from build123d import *

# Parameters (mm, degrees)
SKETCH2_R           = 4
SKETCH2_R_2         = 1.5
BOSS_EXTRUDE1_DEPTH = 5


with BuildPart() as part:
    # Sketch2 → Boss-Extrude1 (new body)
    with BuildSketch(Plane(origin=(0, 0, 0), x_dir=(1, 0, 0), z_dir=(0, 1, 0))):
        with BuildLine():
            ThreePointArc((76.95, 3.434748899), (43.7, -20.636504604), (10.45, 3.434748899))
            ThreePointArc((10.45, 3.434748899), (-3.607827445, 10.391514862), (-10.330163324, -3.779910806))
            ThreePointArc((-10.330163324, -3.779910806), (13.672960294, -33.698499541), (50.894326472, -42.963584275))
            ThreePointArc((50.894326472, -42.963584275), (51.441931195, -42.905082963), (51.985921637, -42.819247444))
            ThreePointArc((51.985921637, -42.819247444), (80.160934451, -29.394967139), (97.781840004, -3.635573974))
            ThreePointArc((97.781840004, -3.635573974), (90.935325704, 10.416403994), (76.95, 3.434748899))
        make_face()
        with Locations((50, -32)):
            Circle(SKETCH2_R, mode=Mode.SUBTRACT)
        Circle(SKETCH2_R_2, mode=Mode.SUBTRACT)
        with Locations((87.4, 0)):
            Circle(SKETCH2_R_2, mode=Mode.SUBTRACT)
    extrude(amount=BOSS_EXTRUDE1_DEPTH)


solid = part.part
Read the model definition and answer for the solid it produces. Units are mm, in the model's axes. Give positions to 0.01 mm unless a question says otherwise; leave off trailing zeros. Loops run counter-clockwise (first coordinate to the right, second up) from the corner with the lowest first, then second, coordinate; pieces in that order, holes last. Notation, with made-up numbers: (80, 65) -> (102, 65) arc R25 cw to (102, 103) -> close; hole circle Ø7 at (-13, 22.5). An arc over 180 degrees is marked (long way). Use a Markdown table: item, result.
Q1. Each of these flat-tipped pins is pushed along its axis until it touches: pin 1 (3 mm diameter, centred on y = 1, z = 3, fed in from +X); pin 2 (2 mm diameter, centred on y = 4, z = 21.5, fed in from -X); pin 3 (2 mm diameter, centred on x = 70.5, y = 1, fed in from +Z). Where does it stop, or does it pass through?
Solved:
| item | result |
|---|---|
| pin 1 | stops at x = 98.3 |
| pin 2 | stops at x = -0.95 |
| pin 3 | stops at z = 36.69 |
Q2. Section C-C, the plane x = 47 is taken. Determine the outline of the cut face in (y, z), then the cut area to 3 significant figures.
Solved:
| item | result |
|---|---|
| outline | (0, 20.48) -> (5, 20.48) -> (5, 29.35) -> (0, 29.35) -> close; (0, 34.65) -> (5, 34.65) -> (5, 43.15) -> (0, 43.15) -> close |
| area | 86.9 mm^2 |
Q3. Section D-D, the plane z = 0 is taken. Determine the outline of the cut face in (x, y).
Solved:
| item | result |
|---|---|
| outline | (-11, 0) -> (-1.5, 0) -> (-1.5, 5) -> (-11, 5) -> close; (1.5, 0) -> (11.78, 0) -> (11.78, 5) -> (1.5, 5) -> close; (75.62, 0) -> (85.9, 0) -> (85.9, 5) -> (75.62, 5) -> close; (88.9, 0) -> (98.4, 0) -> (98.4, 5) -> (88.9, 5) -> close |
Q4. Find the intervals of material crossed by line 1 along X through (y, z) = (0.3, -0.5); line 2 along Z through (x, y) = (51, 2.2); line 3 along Z through (x, y) = (0, 2.7), in increasing order.
Solved:
| item | result |
|---|---|
| line 1 | x = -10.99 to -1.41, 1.41 to 11.56, 75.84 to 85.99, 88.81 to 98.39 |
| line 2 | z = 19.87 to 28.13, 35.87 to 42.95 |
| line 3 | z = -11 to -1.5, 1.5 to 21.67 |
Q5. Determine the mould class of faces 1 (the face through (43, 0, 22)), 2 (the face through (85.9, 2.46, -0.07)), 3 (the face through (79.8, 2.5, 29.7)), 4 (the face through (-1.5, 2.46, -0.07)) for opening direction X: pulls with the +X half, pulls with the -X half, needs draft (parallel to the pull), parting line crosses it, or undercut.
Solved:
| item | result |
|---|---|
| face 1 | needs draft |
| face 2 | undercut |
| face 3 | pulls with the +X half |
| face 4 | undercut |
Q6. Section A-A, the plane y = 3.35 is taken. Determine the outline of the cut face in (x, z), then the cut area to 3 significant figures.
Solved:
| item | result |
|---|---|
| outline | (-10.33, 3.78) arc R11 ccw (long way) to (10.45, -3.43) arc R35 cw to (76.95, -3.43) arc R11 ccw (long way) to (97.78, 3.64) arc R60 ccw to (51.99, 42.82) arc R11 ccw to (50.89, 42.96) arc R60 ccw to start; hole circle Ø3 at (0, 0); hole circle Ø8 at (50, 32); hole circle Ø3 at (87.4, 0) |
| area | 2,850 mm^2 |
Q7. Section B-B, the plane z = 8 is taken. Determine the outline of the cut face in (x, y).
Solved:
| item | result |
|---|---|
| outline | (-8.6, 0) -> (16.78, 0) -> (16.78, 5) -> (-8.6, 5) -> close; (70.62, 0) -> (96.06, 0) -> (96.06, 5) -> (70.62, 5) -> close |
